Autodesk Inventor part; units mm, degrees
ref_plane "YZ Plane" through (0, 0, 0) normal (1, 0, 0) x (0, 1, 0)
ref_plane "XZ Plane" through (0, 0, 0) normal (0, 1, 0) x (-1, 0, 0)
ref_plane "XY Plane" through (0, 0, 0) normal (0, 0, 1) x (1, 0, 0)
sketch "Sketch1" plane through (0, 0, 0) normal (1, 0, 0) x (0, 1, 0)
  line L0 (0, 0) -> (71.5, 0)
  line L1 (71.5, 0) -> (71.5, -83.8)
  line L2 (71.5, -83.8) -> (0, -83.8)
  line L3 (0, -83.8) -> (0, 0)
  dimension "d0" = 83.8
  dimension "d1" = 71.5
extrude "Extrusion1" add sketch "Sketch1" along normal blind 24
fillet "Fillet1" radius 2 4 edges at (24, 71.5, -41.9) (0, 71.5, -41.9) (24, 0, -41.9) (0, 0, -41.9)
sketch "Sketch4" plane through (24, 0, 0) normal (1, 0, 0) x (0, 0, -1)
  line L0 (0, 0) -> (83.8, 0)
  line L1 (0, 69.5) -> (0, 2)
  point P0 (29, 20)
  point P1 (29, 50)
  dimension "d22" = 20
  dimension "d23" = 50
  dimension "d24" = 29
hole "Hole3" at (24, 20, -29) at (24, 50, -29) direction (-1, 0, 0) diameter 2.459 depth 6
properties part number "Meinberg_Box"
The model under review builds one solid part; all positions refer to its coordinate system, in mm. A direction names the side the tool comes from. Round coordinates to 2 decimals unless told otherwise and drop trailing zeros. Order: outer loops, then holes, each group sorted by start corner. A loop starts at its lowest first (then second) coordinate and runs counter-clockwise, first axis right, second up. Notation, with made-up numbers: (82, 39) -> (93, 39) arc R21 ccw to (93, 65) -> close; hole circle Ø10 at (70, -1). An arc over 180 degrees is marked (long way). Return JSON: item names as keys, results as strings.
1. For faces 1 (the face through (20.96, 21.2, -28.73)), 2 (the face through (23.4, 0.57, -41.31)), list the 3-axis set-ups (+Z, -Z, +X, -X, +Y, -Y) from which the entire face can be reached by the end or side of a thin tool; tool diameter is ignored.
Answer block:
{"face 1": "+X", "face 2": "+Z, -Z, +X, -Y"}
2. For L1, parallel to Y at x = 20.25, z = -29; L2, parallel to Y at x = 22.5, z = -29; L3, parallel to Z at x = 22.55, y = 50, list the stretches that pass through material, from the lowest coordinate up. Write a range as [from, to].
Answer block:
{"L1": "y = [0, 18.77], [21.23, 48.77], [51.23, 71.5]", "L2": "y = [0.06, 18.77], [21.23, 48.77], [51.23, 71.44]", "L3": "z = [-83.8, -30.23], [-27.77, 0]"}
3. The part is to be moulded in two halves that separate along Y. For faces 3 (the face through (18, 50, -29)), 4 (the face through (0.57, 0.6, -41.31)), 5 (the face through (12, 71.5, -41)), say which applies: +Y half, -Y half, draft (parallel to the pull), parting line (faces both ways), or undercut.
Answer block:
{"face 3": "undercut", "face 4": "-Y half", "face 5": "+Y half"}
4. Take a section at A-A (z = -29). Write out the cut boundary in (x, y), then the cut area to 3 significant figures.
Answer block:
{"outline": "(0, 2) arc R2 ccw to (2, 0) -> (22, 0) arc R2 ccw to (24, 2) -> (24, 18.77) -> (18, 18.77) -> (18, 21.23) -> (24, 21.23) -> (24, 48.77) -> (18, 48.77) -> (18, 51.23) -> (24, 51.23) -> (24, 69.5) arc R2 ccw to (22, 71.5) -> (2, 71.5) arc R2 ccw to (0, 69.5) -> close", "area": "1,680 mm²"}
